Source: CAD feature listing. Evaluate the final solid. Frame: model axes, mm. Face numbers are marked on the shaded views. A direction names the side the tool comes from. Coordinates: 2 decimals unless noted, no trailing zeros. Write item = value, one per line. Start each with the question number.
1. Access query for the marked faces 4, 5, 6 and 7. Directions: +Z, -Z, +X, -X, +Y, -Y. A direction counts if a zero-diameter tool reaches every point of the face in a straight line with its end or side. Return the directions, or none.
2. Section query A-A (z = 0). Give the number of separate pieces and of enclosed holes in the cut face, then the cut area to 3 significant figures.
3. Pull-direction query (X, two-part tool) for the marked faces 1, 2 and 3; classes: pulls with the +X half, pulls with the -X half, needs draft (parallel to the pull), parting line crosses it, or undercut.
4. Line query: line 1 along Y through (x, z) = (-225, 0); line 2 along Y through (x, z) = (8, -40); line 3 along X through (y, z) = (48.5, -127). Output: solid intervals per line, ascending.
5. Pin query (flat end, axial travel): pin 1 Ø14.5 at (y, z) = (-80.82, 80.82) entering from -X; pin 2 Ø1.5 at (y, z) = (137, -140) entering from +X; pin 3 Ø6 at (x, y) = (-83, -71) entering from -Z. Return the tip coordinate at first contact, or that it passes through.
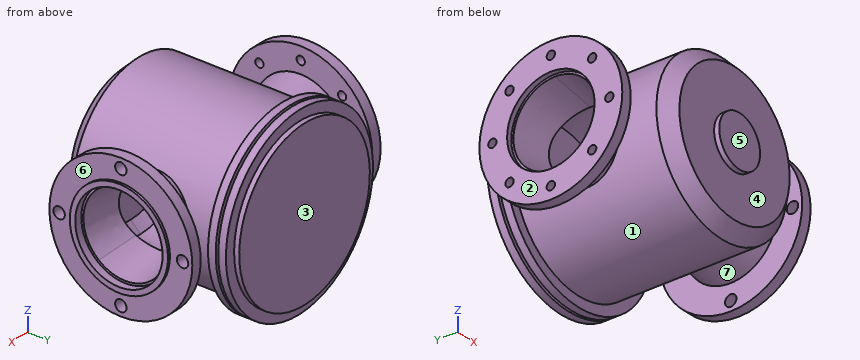
```python
from build123d import *

# Parameters (mm, degrees)
SKETCH2_W                   = 20
SKETCH2_H                   = 15
SHELL1_START                = -39.5000001
SHELL1_OUTLINE_R            = 85.5
SHELL1_DEPTH                = 79.0000001
SHELL1_START_2              = -235.4
SHELL1_2_OUTLINE_R          = 85.5
SHELL1_2_DEPTH              = 14.9
SHELL1_START_3              = 220.5
SHELL1_3_OUTLINE_R          = 85.5
SHELL1_3_DEPTH              = 14.9
SHELL1_START_4              = -145.650757695
SHELL1_4_OUTLINE_R          = 149.5
SHELL1_4_DEPTH              = 310.150757695
SHELL1_START_5              = -174.5
SHELL1_5_OUTLINE_R          = 39.5
SHELL1_5_DEPTH              = 89
CUT_EXTRUDE1_REACH          = 534.755
SKETCH5_R                   = 11.175
CIRPATTERN1_COUNT           = 4
SKETCH15_R                  = 96
CUT_EXTRUDE4_DEPTH          = 4.75
SKETCH14_R                  = 39.5
EXTRUDE2_DEPTH              = 10
F_5_8_CLEARANCE_HOLE5_D     = 16.27124
F_5_8_CLEARANCE_HOLE5_DEPTH = 20.65


with BuildPart() as part:
    # Sketch1 → Base-Revolve (revolve)
    with BuildSketch(Plane.XY, mode=Mode.PRIVATE) as base_revolve_sk:
        Polygon((0, -185), (50, -185), (50, -175), (135, -175), (160, -150), (160, 175), (0, 175), align=None)
    revolve(base_revolve_sk.sketch.rotate(Axis((0, -64.079408138, 0), (0, 1, 0)), 90), axis=Axis((0, -64.079408138, 0), (0, 1, 0)))

    # Sketch2 → Boss-Revolve1 (revolve)
    with BuildSketch(Plane.XY, mode=Mode.PRIVATE) as boss_revolve1_sk:
        with Locations((170, 157.5)):
            Rectangle(SKETCH2_W, SKETCH2_H)
        with Locations((170, 137.5)):
            Rectangle(SKETCH2_W, SKETCH2_H)
    revolve(boss_revolve1_sk.sketch.rotate(Axis((0, 0, 0), (0, 1, 0)), 90), axis=Axis((0, 0, 0), (0, 1, 0)))

    # Sketch3 → Boss-Revolve2 (revolve)
    with BuildSketch(Plane.XY, mode=Mode.PRIVATE) as boss_revolve2_sk:
        Polygon((0, 0), (0, 52.971334051), (210, 90), (210, 139.7), (230.65, 139.7), (230.65, 96), (235.4, 96), (235.4, 0), align=None)
    boss_revolve2 = revolve(boss_revolve2_sk.sketch.rotate(Axis((0, 0, 0), (1, 0, 0)), 90), axis=Axis((0, 0, 0), (1, 0, 0)))

    # Mirror1: Boss-Revolve2 across plane
    add(boss_revolve2.mirror(Plane(origin=(0, 0, 0), x_dir=(0, 0, 1), z_dir=(1, 0, 0))))

    # Shell1: read off the stored shape, not the designer's step
    # Shell1 outline → Shell1 (cut)
    with BuildSketch(Plane.YZ.offset(SHELL1_START)):
        Circle(SHELL1_OUTLINE_R)
    extrude(amount=SHELL1_DEPTH, mode=Mode.SUBTRACT)

    # Shell1 2 outline → Shell1 2 (cut)
    with BuildSketch(Plane.YZ.offset(SHELL1_START_2)):
        Circle(SHELL1_2_OUTLINE_R)
    extrude(amount=SHELL1_2_DEPTH, mode=Mode.SUBTRACT)

    # Shell1 3 outline → Shell1 3 (cut)
    with BuildSketch(Plane.YZ.offset(SHELL1_START_3)):
        Circle(SHELL1_3_OUTLINE_R)
    extrude(amount=SHELL1_3_DEPTH, mode=Mode.SUBTRACT)

    # Shell1 4 outline → Shell1 4 (cut)
    with BuildSketch(Plane(origin=(0, 0, 0), x_dir=(1, 0, 0), z_dir=(0, 1, 0)).offset(SHELL1_START_4)):
        Circle(SHELL1_4_OUTLINE_R)
    extrude(amount=SHELL1_4_DEPTH, mode=Mode.SUBTRACT)

    # Shell1 5 outline → Shell1 5 (cut)
    with BuildSketch(Plane(origin=(0, 0, 0), x_dir=(1, 0, 0), z_dir=(0, 1, 0)).offset(SHELL1_START_5)):
        Circle(SHELL1_5_OUTLINE_R)
    extrude(amount=SHELL1_5_DEPTH, mode=Mode.SUBTRACT)

    # Shell1 6: loft between two sections, ruled curve by curve
    shell1_6_from = [
        Edge.make_three_point_arc((0, -164.5, 130.650757595), (130.650757595, -164.5, 0), (0, -164.5, -130.650757595)),
        Edge.make_three_point_arc((0, -164.5, -130.650757595), (-130.650757595, -164.5, 0), (0, -164.5, 130.650757595)),
    ]
    shell1_6_to = [
        Edge.make_three_point_arc((0, -145.650757595, 149.5), (149.5, -145.650757595, 0), (0, -145.650757595, -149.5)),
        Edge.make_three_point_arc((0, -145.650757595, -149.5), (-149.5, -145.650757595, 0), (0, -145.650757595, 149.5)),
    ]
    shell1_6 = Solid(Shell([*[Face.make_surface_from_curves(shell1_6_from[k], shell1_6_to[k]) for k in range(2)], Face(Wire(shell1_6_from)), Face(Wire(shell1_6_to))]))
    add(shell1_6, mode=Mode.SUBTRACT)

    # Shell1 7: loft between two sections, ruled curve by curve
    shell1_7_from = [
        Edge.make_three_point_arc((134.158642782, 41.530655606, 51.250412113), (134.158642782, -51.250412113, 41.530655606), (134.158642782, -41.530655606, -51.250412113)),
        Edge.make_three_point_arc((134.158642782, -41.530655606, -51.250412113), (134.158642782, 51.250412113, -41.530655606), (134.158642782, 41.530655606, 51.250412113)),
    ]
    shell1_7_to = [
        Edge.make_three_point_arc((220.5, 51.115651267, 63.078662127), (220.5, -63.078662127, 51.115651267), (220.5, -51.115651267, -63.078662127)),
        Edge.make_three_point_arc((220.5, -51.115651267, -63.078662127), (220.5, 63.078662127, -51.115651267), (220.5, 51.115651267, 63.078662127)),
    ]
    shell1_7 = Solid(Shell([*[Face.make_surface_from_curves(shell1_7_from[k], shell1_7_to[k]) for k in range(2)], Face(Wire(shell1_7_from)), Face(Wire(shell1_7_to))]))
    add(shell1_7, mode=Mode.SUBTRACT)

    # Shell1 8: loft between two sections, ruled curve by curve
    shell1_8_from = [
        Edge.make_three_point_arc((-134.158707207, 0, -65.965154404), (-134.158707207, -65.965154404, 0), (-134.158707207, 0, 65.965154404)),
        Edge.make_three_point_arc((-134.158707207, 0, 65.965154404), (-134.158707207, 65.965154404, 0), (-134.158707207, 0, -65.965154404)),
    ]
    shell1_8_to = [
        Edge.make_three_point_arc((-220.5, 0, -81.189453873), (-220.5, -81.189453873, 0), (-220.5, 0, 81.189453873)),
        Edge.make_three_point_arc((-220.5, 0, 81.189453873), (-220.5, 81.189453873, 0), (-220.5, 0, -81.189453873)),
    ]
    shell1_8 = Solid(Shell([*[Face.make_surface_from_curves(shell1_8_from[k], shell1_8_to[k]) for k in range(2)], Face(Wire(shell1_8_from)), Face(Wire(shell1_8_to))]))
    add(shell1_8, mode=Mode.SUBTRACT)

    # Sketch5 → Cut-Extrude1 (cut, up to next)
    with BuildSketch(Plane(origin=(230.65, 0, 0), x_dir=(0, 0, -1), z_dir=(1, 0, 0)), mode=Mode.PRIVATE) as cut_extrude1_sk1:
        with Locations((0, 120.65)):
            Circle(SKETCH5_R)
    cut_extrude1_tool1 = extrude(cut_extrude1_sk1.sketch, amount=-CUT_EXTRUDE1_REACH, mode=Mode.PRIVATE) & part.part
    cut_extrude1 = cut_extrude1_tool1.solids().sort_by_distance((230.65, 120.65, 0))[0]
    add(cut_extrude1, mode=Mode.SUBTRACT)

    # CirPattern1: Cut-Extrude1 ×4 about axis
    cirpattern1_axis = Axis((0, 0, 0), (1, 0, 0))
    for i in range(1, CIRPATTERN1_COUNT):
        add(cut_extrude1.rotate(cirpattern1_axis, i * 360 / CIRPATTERN1_COUNT), mode=Mode.SUBTRACT)

    # Sketch15 → Cut-Extrude4 (cut)
    with BuildSketch(Plane.ZY.offset(230.65)):
        Circle(SKETCH15_R)
    extrude(amount=CUT_EXTRUDE4_DEPTH, mode=Mode.SUBTRACT)

    # Sketch14 → Extrude2 (add)
    with BuildSketch(Plane(origin=(0, -174.5, 0), x_dir=(1, 0, 0), z_dir=(0, 1, 0))):
        Circle(SKETCH14_R)
    extrude(amount=EXTRUDE2_DEPTH)

    # 5/8 Clearance Hole5
    with Locations(Plane(origin=(-230.65, -86.94526051, 61.229912904), x_dir=(0, 0, 1), z_dir=(-1, 0, 0))):
        with Locations((-61.229912904, 201.24526051), (-176.596487394, 86.94526051), (-142.052217993, 167.767565599), (19.592392186, 167.767565599), (53.070087096, 86.94526051), (19.592392186, 6.12295542), (-61.229912904, -27.406492985), (-142.052217993, 6.12295542)):
            Hole(F_5_8_CLEARANCE_HOLE5_D / 2, depth=F_5_8_CLEARANCE_HOLE5_DEPTH)


solid = part.part
```
Results are:
q1.face_4 = -Y
q1.face_5 = +Z, -Z, +X, -X, -Y
q1.face_6 = +X
q1.face_7 = none
q2.separate_pieces = 6
q2.enclosed_holes = 0
q2.area = 18,000 mm^2
q3.face_1 = undercut
q3.face_2 = pulls with the -X half
q3.face_3 = needs draft
q4.line_1 = -139.7 to -122.49, -106.22 to -85.5, 85.5 to 106.16, 122.44 to 139.7
q4.line_2 = -185 to -164.5, 164.5 to 175
q4.line_3 = -230.65 to -210, -97.32 to -78.87, 78.87 to 97.32, 210 to 230.65
q5.pin_1 = -142.08
q5.pin_2 = 114.06
q5.pin_3 = -138.56
